from build123d import *

# Parameters (mm, degrees)
BOSS_EXTRUDE1_DEPTH = 5.9944
BOSS_EXTRUDE2_DEPTH = 4.318
BOSS_EXTRUDE3_DEPTH = 3.048
CIRPATTERN1_COUNT   = 21
SKETCH4_R           = 0.9
CUT_EXTRUDE1_DEPTH  = 6
CUT_EXTRUDE2_REACH  = 35.989


with BuildPart() as part:
    # Sketch1 → Boss-Extrude1 (new, symmetric)
    with BuildSketch(Plane(origin=(0, 0, 0), x_dir=(0, 0, -1), z_dir=(1, 0, 0))):
        Polygon((22.45, 16.764), (27.325, 16.764), (27.325, 19.304), (22.45, 19.304), (22.45, 22.479), (0, 22.479), (0, 19.304), (-4.875, 19.304), (-4.875, 16.764), (0, 16.764), (0, 0), (22.45, 0), align=None)
    extrude(amount=BOSS_EXTRUDE1_DEPTH, both=True)

    # Sketch2 → Boss-Extrude2 (add)
    with BuildSketch(Plane(origin=(0, 22.479, 0), x_dir=(1, 0, 0), z_dir=(0, 1, 0))):
        with BuildLine():
            ThreePointArc((-2.717065955, 11.337655932), (0, 0), (2.717065955, 11.337655932))
            ThreePointArc((2.717065955, 11.337655932), (0, 14.7828), (-2.717065955, 11.337655932))
        make_face()
    extrude(amount=BOSS_EXTRUDE2_DEPTH)

    # Sketch3 → Boss-Extrude3 (add)
    with BuildSketch(Plane(origin=(0, 26.797, 0), x_dir=(1, 0, 0), z_dir=(0, 1, 0))):
        Polygon((0, 5.9944), (0, 8.3058), (0.363424662, 8.405565087), (0.68129711, 8.203110983), align=None)
    boss_extrude3 = extrude(amount=BOSS_EXTRUDE3_DEPTH)

    # CirPattern1: Boss-Extrude3 ×21 about axis
    cirpattern1_axis = Axis((0, 0, -5.9944), (0, 1, 0))
    for i in range(1, CIRPATTERN1_COUNT):
        add(boss_extrude3.rotate(cirpattern1_axis, i * 360 / CIRPATTERN1_COUNT))

    # Sketch4 → Cut-Extrude1 (cut)
    with BuildSketch(Plane(origin=(0, 29.845, 0), x_dir=(1, 0, 0), z_dir=(0, 1, 0))):
        with Locations(Location((0, 5.9944, 0), (0, 0, 270))):
            Circle(SKETCH4_R)
    extrude(amount=-CUT_EXTRUDE1_DEPTH, mode=Mode.SUBTRACT)

    # Sketch5 → Cut-Extrude2 (cut, up to next)
    with BuildSketch(Plane(origin=(0, 19.304, 0), x_dir=(1, 0, 0), z_dir=(0, 1, 0)), mode=Mode.PRIVATE) as cut_extrude2_sk1:
        with BuildLine():
            Line((-0.6096, 26.054950376), (-0.6096, 27.325))
            Line((-0.6096, 27.325), (0.6096, 27.325))
            Line((0.6096, 27.325), (0.6096, 26.054950376))
            ThreePointArc((0.6096, 26.054950376), (0, 24.1409), (-0.6096, 26.054950376))
        make_face()
    cut_extrude2_tool1 = extrude(cut_extrude2_sk1.sketch, amount=-CUT_EXTRUDE2_REACH, mode=Mode.PRIVATE) & part.part
    # Sketch5 → Cut-Extrude2 (cut, up to next)
    with BuildSketch(Plane(origin=(0, 19.304, 0), x_dir=(1, 0, 0), z_dir=(0, 1, 0)), mode=Mode.PRIVATE) as cut_extrude2_sk2:
        with BuildLine():
            Line((-0.6096, -4.875), (0.6096, -4.875))
            Line((0.6096, -4.875), (0.6096, -3.604950376))
            ThreePointArc((0.6096, -3.604950376), (0, -1.6909), (-0.6096, -3.604950376))
            Line((-0.6096, -3.604950376), (-0.6096, -4.875))
        make_face()
    cut_extrude2_tool2 = extrude(cut_extrude2_sk2.sketch, amount=-CUT_EXTRUDE2_REACH, mode=Mode.PRIVATE) & part.part
    add(cut_extrude2_tool1.solids().sort_by_distance((0, 19.304, -25.638579))[0], mode=Mode.SUBTRACT)
    add(cut_extrude2_tool2.solids().sort_by_distance((0, 19.304, 3.188579))[0], mode=Mode.SUBTRACT)


solid = part.part
Verification items for the finished model (mm, model axes). A direction names the side the tool comes from. Round coordinates to 2 decimals unless told otherwise and drop trailing zeros. Loops run counter-clockwise (first coordinate to the right, second up) from the corner with the lowest first, then second, coordinate; pieces in that order, holes last. Notation, with made-up numbers: (-8, 48) - (2, 48) arc R29 cw to (2, 76) - close; hole circle Ø2 at (-29.75, 39). An arc over 180 degrees is marked (long way). Use a Markdown table: item, result. Add a question column.
1. Thickness scan on probe 1 along Y at (x, z) = (3.25, -10.5); probe 2 along Y at (x, z) = (-5, -16); probe 3 along Z at (x, y) = (4.25, 15). Record the ranges inside material, lowest first. Write a range as [from, to].
2. Access from +Z, -Z, +X, -X, +Y, -Y to the whole of each face (thin tool, end or side, straight path). Record for faces 5 (the face through (0, 26.797, -9)), 6 (the face through (-5, 22.479, -1)), 7 (the face through (0.1, 16.764, -23.8)).
3. Section check A-A, the plane x = 4. Record the boundary of the cut face in (y, z) (3 decimals), plus the area to 3 significant figures.
4. Release check for a two-part mould opening along Z. For faces 1 (the face through (0, 8, 0)), 2 (the face through (0, 0, -11)), 3 (the face through (3, 18, -27.325)), 4 (the face through (0, 23.845, -6)) record: released by +Z, released by -Z, zero draft, split by the parting line, or undercut.
5. Section check B-B, the plane z = -17. Record the boundary of the cut face in (x, y), plus the area to 3 significant figures.
6. Section check C-C, the plane y = 15. Record the boundary of the cut face in (x, z).
7. Section check D-D, the plane x = -3.5. Record the boundary of the cut face in (y, z) (3 decimals), plus the area to 3 significant figures.
8. Gauge pin test, flat ends, axial feed: pin 1 (4 mm diameter, centred on x = 1.5, z = -25, fed in from +Y); pin 2 (1.9 mm diameter, centred on x = 0, z = 2.745, fed in from -Y); pin 3 (1.5 mm diameter, centred on x = -2, y = 14.5, fed in from +Z); pin 4 (1 mm diameter, centred on x = 1.5, y = 20.5, fed in from -Z). Record the tip position at first contact, or that the pin passes through.
Checks:
| question | item | result |
|---|---|---|
| 1 | probe 1 | y = [0, 26.8] |
| 1 | probe 2 | y = [0, 22.48] |
| 1 | probe 3 | z = [-22.45, 0] |
| 2 | face 5 | +Y |
| 2 | face 6 | +Z, -X, +Y |
| 2 | face 7 | -Z, +X, -X, -Y |
| 3 | outline | (0, -22.45) - (16.764, -22.45) - (16.764, -27.325) - (19.304, -27.325) - (19.304, -22.45) - (22.479, -22.45) - (22.479, -10.459) - (26.797, -10.459) - (26.797, -1.53) - (22.479, -1.53) - (22.479, 0) - (19.304, 0) - (19.304, 4.875) - (16.764, 4.875) - (16.764, 0) - (0, 0) - close |
| 3 | area | 568 mm^2 |
| 4 | face 1 | released by +Z |
| 4 | face 2 | zero draft |
| 4 | face 3 | released by -Z |
| 4 | face 4 | undercut |
| 5 | outline | (-5.99, 0) - (5.99, 0) - (5.99, 22.48) - (-5.99, 22.48) - close |
| 5 | area | 269 mm^2 |
| 6 | outline | (-5.99, -22.45) - (5.99, -22.45) - (5.99, 0) - (-5.99, 0) - close |
| 7 | outline | (0, -22.45) - (16.764, -22.45) - (16.764, -27.325) - (19.304, -27.325) - (19.304, -22.45) - (22.479, -22.45) - (22.479, -10.861) - (26.797, -10.861) - (26.797, -1.128) - (22.479, -1.128) - (22.479, 0) - (19.304, 0) - (19.304, 4.875) - (16.764, 4.875) - (16.764, 0) - (0, 0) - close |
| 7 | area | 571 mm^2 |
| 8 | pin 1 | stops at y = 19.3 |
| 8 | pin 2 | passes through |
| 8 | pin 3 | stops at z = 0 |
| 8 | pin 4 | stops at z = -22.45 |
